from build123d import *

# Parameters (mm, degrees)
EXTRUDE_1_DEPTH     = 12
SKETCH_2_R          = 8
CUT_EXTRUDE_1_DEPTH = 8
SKETCH_3_R          = 2.5
CUT_EXTRUDE_2_DEPTH = 10


with BuildPart() as part:
    # 草图1 → 凸台-拉伸1 (new body)
    with BuildSketch(Plane(origin=(0, 0, 0), x_dir=(0, 0, -1), z_dir=(1, 0, 0))):
        with BuildLine():
            Line((-22.5, 15), (22.5, 15))
            ThreePointArc((22.5, 15), (26.035533906, 13.535533906), (27.5, 10))
            Line((27.5, 10), (27.5, -10))
            ThreePointArc((27.5, -10), (26.035533906, -13.535533906), (22.5, -15))
            Line((22.5, -15), (-22.5, -15))
            ThreePointArc((-22.5, -15), (-26.035533906, -13.535533906), (-27.5, -10))
            Line((-27.5, -10), (-27.5, 10))
            ThreePointArc((-27.5, 10), (-26.035533906, 13.535533906), (-22.5, 15))
        make_face()
    extrude(amount=EXTRUDE_1_DEPTH)

    # 草图2 → 切除-拉伸1 (cut)
    with BuildSketch(Plane.ZY):
        Circle(SKETCH_2_R)
    extrude(amount=-CUT_EXTRUDE_1_DEPTH, mode=Mode.SUBTRACT)

    # 草图3 → 切除-拉伸2 (cut)
    with BuildSketch(Plane.XZ.offset(15)):
        with Locations((3, 0)):
            Circle(SKETCH_3_R)
    extrude(amount=-CUT_EXTRUDE_2_DEPTH, mode=Mode.SUBTRACT)


solid = part.part
For this review, take the finished solid that the model builds, in its own axes (mm). A direction names the side the tool comes from. Round coordinates to 2 decimals unless told otherwise and drop trailing zeros. Order: outer loops, then holes, each group sorted by start corner. A loop starts at its lowest first (then second) coordinate and runs counter-clockwise, first axis right, second up. Notation, with made-up numbers: (-34, -1.75) -> (12, -1.75) arc R20 cw to (12, 20.25) -> close; hole circle Ø10 at (43, 86). An arc over 180 degrees is marked (long way). Put each result on its own line as item: value.
Q1. Insertion check: pin 1 Ø4 at (x, y) = (8, -12) entering from -Z; pin 2 Ø9.5 at (y, z) = (0, 0) entering from -X. Each pin has a flat end and moves straight along its axis. Give the tip position at first contact, or say it passes through.
Check result:
pin 1: z = -27.5
pin 2: x = 8
Q2. Machinability: for faces 5 (the cylindrical face through (5.92, 13.5, 26.07)), 6 (the cylindrical face through (3.944, 6.746, 4.301)), which of the approach directions +Z, -Z, +X, -X, +Y, -Y give a long, thin tool a straight path to every point of the face, cutting with its end or side? Answer none if there is none.
Check result:
face 5: +Z, +X, -X, +Y
face 6: -X
Q3. For probe 1 along Y at (x, z) = (6.75, 0); probe 2 along X at (y, z) = (-11, 0); probe 3 along X at (y, z) = (-1, -4.5), list the stretches that pass through material, from the lowest coordinate up. Write a range as [from, to].
Check result:
probe 1: [-15, -8], [8, 15]
probe 2: [0, 0.5], [5.5, 12]
probe 3: [8, 12]
Q4. Add section D-D on y = 0. Write out the cut boundary in (x, z).
Check result:
outline: (0, -27.5) -> (12, -27.5) -> (12, 27.5) -> (0, 27.5) -> (0, 8) -> (8, 8) -> (8, -8) -> (0, -8) -> close
Q5. Add section C-C on x = 3. Write out the cut boundary in (y, z).
Check result:
outline: (-15, -22.5) arc R5 ccw to (-10, -27.5) -> (10, -27.5) arc R5 ccw to (15, -22.5) -> (15, 22.5) arc R5 ccw to (10, 27.5) -> (-10, 27.5) arc R5 ccw to (-15, 22.5) -> (-15, 2.5) -> (-7.6, 2.5) arc R8 cw (long way) to (-7.6, -2.5) -> (-15, -2.5) -> close
Q6. Add section B-B on z = 0. Write out the cut boundary in (x, y), plus the area to 3 significant figures.
Check result:
outline: (0, -15) -> (0.5, -15) -> (0.5, -8) -> (0, -8) -> close; (0, 8) -> (8, 8) -> (8, -8) -> (5.5, -8) -> (5.5, -15) -> (12, -15) -> (12, 15) -> (0, 15) -> close
area: 197 mm2
Q7. Mouldability with a two-part tool opening along X and no side actions: class faces 1 (the cylindrical face through (5.92, -13.57, 26)), 2 (the flat face through (0, 7, -6)), 3 (the flat face through (12, 0, 0)), 4 (the cylindrical face through (1, -11.3, -1.5)) as pulls with the +X half, pulls with the -X half, needs draft (parallel to the pull), parting line crosses it, or undercut.
Check result:
face 1: needs draft
face 2: pulls with the -X half
face 3: pulls with the +X half
face 4: undercut
Q8. Add section A-A on y = -9. Write out the cut boundary in (x, z).
Check result:
outline: (0, -27.5) -> (12, -27.5) -> (12, 27.5) -> (0, 27.5) -> close; hole circle Ø5 at (3, 0)
